```python
from build123d import *

# Parameters (mm, degrees)
F0_R        = 106.68
F1_DEPTH    = 50
F2_R        = 9
F4_W        = 88.5786805532
F4_H        = 25.534863025
F5_DEPTH    = 100
F6_T        = 2.54
F6_T3_DEPTH = 30.08
F6_T5_DEPTH = 10.8915489546
F6_T7_DEPTH = 205.08
F6_T9_DEPTH = 10.8915489546


# Not quite as in the source:
# - a shell that OpenCascade refuses in one call is made with other operations: the cavity is built on its own and cut out


with BuildPart() as f1:
    # F0 (on Top) → F1 (new body)
    with BuildSketch(Plane.XY):
        Circle(F0_R)
    extrude(amount=F1_DEPTH)

    # F2 (on Front) → F3 (revolve, cut)
    with BuildSketch(Plane.XZ):
        with Locations((41.004, 0)):
            Circle(F2_R)
    revolve(axis=Axis((0, 0, 20.5781124532), (0, 0, 1)), mode=Mode.SUBTRACT)

    # F4 (on Right) → F5 (cut, symmetric)
    with BuildSketch(Plane.YZ):
        with Locations((75.6345188421, 37.7674315125)):
            Rectangle(F4_W, F4_H)
        with Locations((-75.6345188421, 37.7674315125)):
            Rectangle(F4_W, F4_H)
    extrude(amount=F5_DEPTH, both=True, mode=Mode.SUBTRACT)

    # F6: shell of thickness 2.54, made by hand


with BuildPart() as f6_core1:
    # F6_t2: copy of F1
    add(f1.part)

    # the walls: a layer under each face that stays
    f6_faces = [f6_core1.faces().sort_by_distance(p)[0] for p in [
        (-106.68, 0, 25),
        (-71.12, -71.12, 0),
        (100, -34.2509530428, 37.5),
        (0, -69.0125892827, 25),
        (-100, -34.2509530428, 37.5),
        (-100, 34.2509530428, 37.5),
        (0, 69.0125892827, 25),
        (100, 34.2509530428, 37.5),
        (-41.004, 0, 9),
        (0, -31.3451785655, 37.5),
        (0, 31.3451785655, 37.5),
        (0, 0, 0),
    ]]
    thicken(f6_faces, amount=-F6_T, mode=Mode.SUBTRACT)

    # F6_s4 → F6_t3 (cut)
    with BuildSketch(Plane.XY.offset(22.46)):
        Polygon((99.9746, -31.3705785655), (102.54, -31.3451785655), (102.54, -28.8051785655), (100, -28.8051785655), align=None)
        Polygon((-99.9746, -31.3705785655), (-102.54, -31.3451785655), (-102.54, -28.8051785655), (-100, -28.8051785655), align=None)
        Polygon((-99.9746, 31.3705785655), (-102.54, 31.3451785655), (-102.54, 28.8051785655), (-100, 28.8051785655), align=None)
        Polygon((99.9746, 31.3705785655), (102.54, 31.3451785655), (102.54, 28.8051785655), (100, 28.8051785655), align=None)
    extrude(amount=F6_T3_DEPTH, mode=Mode.SUBTRACT)

    # F6_s6 → F6_t5 (cut)
    with BuildSketch(Plane.XZ.offset(28.8051785655)):
        Polygon((99.9746, 25.0254), (102.54, 25), (102.54, 22.46), (100, 22.46), align=None)
        Polygon((-99.9746, 25.0254), (-100, 22.46), (-102.54, 22.46), (-102.54, 25), align=None)
    extrude(amount=F6_T5_DEPTH, mode=Mode.SUBTRACT)

    # F6_s8 → F6_t7 (cut)
    with BuildSketch(Plane.YZ.offset(-102.54)):
        Polygon((-31.3705785655, 25.0254), (-31.3451785655, 22.46), (-28.8051785655, 22.46), (-28.8051785655, 25), align=None)
        Polygon((31.3705785655, 25.0254), (31.3451785655, 22.46), (28.8051785655, 22.46), (28.8051785655, 25), align=None)
    extrude(amount=F6_T7_DEPTH, mode=Mode.SUBTRACT)

    # F6_s10 → F6_t9 (cut)
    with BuildSketch(Plane.XZ.offset(-39.6967275201)):
        Polygon((-99.9746, 25.0254), (-102.54, 25), (-102.54, 22.46), (-100, 22.46), align=None)
        Polygon((99.9746, 25.0254), (100, 22.46), (102.54, 22.46), (102.54, 25), align=None)
    extrude(amount=F6_T9_DEPTH, mode=Mode.SUBTRACT)


with BuildPart() as f1_1:
    add(f1.part)

    # what is left inside the walls is the cavity
    f6_cavity = [f6_core1.part.solids().sort_by_distance(p)[0] for p in [
        (-52.07, 34.713333, 2.5654),
    ]]
    add(f6_cavity, mode=Mode.SUBTRACT)


solid = f1_1.part
```
Build history of the part. All positions in model axes, mm. A direction names the side the tool comes from. Round coordinates to 2 decimals unless told otherwise and drop trailing zeros. Write each loop counter-clockwise with the first axis right and the second up, starting at its lowest first coordinate (ties: lowest second). Pieces come first, ordered by that corner, then holes.
1) 3-axis set-ups, long thin cutter, end or side, ignore diameter. For faces 5 (the flat face through (1, -61, 25)), 6 (the flat face through (-1, 31.345, 37)), 7 (the flat face through (-1, 59, 22.46)): which of +Z, -Z, +X, -X, +Y, -Y reach the whole face in a straight line?
2) Pin check, flat tips, straight feed: pin 1 (6.5 mm diameter, centred on y = 35, z = 36, fed in from +X); pin 2 (3 mm diameter, centred on x = 32.5, z = 34, fed in from -Y); pin 3 (8 mm diameter, centred on y = 22.5, z = 16.5, fed in from +X). Stop position of each tip, or through.
3) Drill centre lines: probe 1 along Y at (x, z) = (0, 21); probe 2 along Z at (x, y) = (-14.5, -57.5); probe 3 along Y at (x, z) = (0, 33.5). Where is each one in solid material? Low to high.
4) Band-saw the part on D-D, the plane y = 0. List the corners of the cut face in (x, z), and give its area (3 significant figures).
5) Band-saw the part on B-B, the plane y = 80.5. List the corners of the cut face in (x, z), and give its area (3 significant figures).
6) Mould opens along X. For faces 1 (the flat face through (0, 0, 0)), 2 (the flat face through (-1, 28.805, 36)), 3 (the cylindrical face through (-13.89, 105.77, 19.09)), 4 (the flat face through (0, 0, 2.54)) say: +X half, -X half, draft (parallel to the pull), parting line (faces both ways), or undercut.
7) Band-saw the part on C-C, the plane x = 0. List the corners of the cut face in (y, z).
8) Band-saw the part on A-A, the plane z = 38.5. List the corners of the cut face in (x, y), and give its area (3 significant figures).
Ans:
1. face 5: +Z, -Y
1. face 6: +Z, +Y
1. face 7: none
2. pin 1: stops at x = 101.85
2. pin 2: stops at y = -31.35
2. pin 3: stops at x = 105.06
3. probe 1: y = -106.68 to -104.14, 104.14 to 106.68
3. probe 2: z = 0 to 2.54, 22.46 to 25
3. probe 3: y = -31.35 to -28.81, 28.81 to 31.35
4. outline: (-106.68, 0) - (-50, 0) arc R9 cw to (-32, 0) - (32, 0) arc R9 cw to (50, 0) - (106.68, 0) - (106.68, 50) - (104.14, 50) - (104.14, 2.54) - (52.26, 2.54) arc R11.54 ccw to (29.75, 2.54) - (-29.75, 2.54) arc R11.54 ccw to (-52.26, 2.54) - (-104.14, 2.54) - (-104.14, 50) - (-106.68, 50) - close
4. area: 831 mm2
5. outline: (-70, 0) - (70, 0) - (70, 25) - (-70, 25) - close; hole (-66.07, 2.54) - (66.07, 2.54) - (66.07, 22.46) - (-66.07, 22.46) - close
5. area: 868 mm2
6. face 1: draft
6. face 2: undercut
6. face 3: parting line
6. face 4: undercut
7. outline: (-106.68, 0) - (-50, 0) arc R9 cw to (-32, 0) - (32, 0) arc R9 cw to (50, 0) - (106.68, 0) - (106.68, 25) - (31.35, 25) - (31.35, 50) - (28.81, 50) - (28.81, 22.46) - (104.14, 22.46) - (104.14, 2.54) - (52.26, 2.54) arc R11.54 ccw to (29.75, 2.54) - (-29.75, 2.54) arc R11.54 ccw to (-52.26, 2.54) - (-104.14, 2.54) - (-104.14, 22.46) - (-28.81, 22.46) - (-28.81, 50) - (-31.35, 50) - (-31.35, 25) - (-106.68, 25) - close
8. outline: (-100, -37.16) - (-100, -31.35) - (100, -31.35) - (100, -37.16) arc R106.68 ccw to (100, 37.16) - (100, 31.35) - (-100, 31.35) - (-100, 37.16) arc R106.68 ccw to start; hole (-100.08, -28.81) - (100.08, -28.81) arc R104.14 ccw to (100.08, 28.81) - (-100.08, 28.81) arc R104.14 ccw to start
8. area: 1,360 mm2
